Design review of the part built by this model. Coordinates are the model's own, in mm. Coordinates: 2 decimals unless noted, no trailing zeros. Write each loop counter-clockwise with the first axis right and the second up, starting at its lowest first coordinate (ties: lowest second). Pieces come first, ordered by that corner, then holes.
Q1. Add section B-B, the plane x = 4.15. Give the boundary of the cut face in (y, z), plus the area to 3 significant figures.
Q2. To check wall thickness, follow probe 1 along Y at (x, z) = (3.6, -4.45); probe 2 along Y at (x, z) = (3.65, -3.4); probe 3 along Z at (x, y) = (4.65, -2.5). State the ranges of each line that lie inside material, in increasing order.
Q3. Add section A-A, the plane z = -5.45. Give the boundary of the cut face in (x, y).
from build123d import *
from build123d import SkipClean  # not in build123d's __all__

# Parameters (mm, degrees)
F0_W     = 6
F0_H     = 6
F1_DEPTH = 3
F3_ANGLE = 180


with BuildPart() as f1:
    # F0 (on Front) → F1 (new body)
    with BuildSketch(Plane.XZ):
        with Locations((3.4017860889, -4.7885723032)):
            Rectangle(F0_W, F0_H)
    extrude(amount=F1_DEPTH)

    # F2 (on face) → F3 (revolve, cut)
    with BuildSketch(Plane.XZ.offset(3)):
        with BuildLine():
            ThreePointArc((3.4017860889, -6.7885723032), (5.4017860889, -4.7885723032), (3.4017860889, -2.7885723032))
            Line((3.4017860889, -2.7885723032), (3.4017860889, -6.7885723032))
        make_face()
    revolve(axis=Axis((3.4017860889, -3, -4.7885723032), (0, 0, 1)), revolution_arc=F3_ANGLE, mode=Mode.SUBTRACT)

    # F4: F1 across face


with BuildPart() as f1_1:
    add(f1.part, clean=False)
    with SkipClean():  # cleaning this boolean's faces spoils the solid; the shape is the same uncleaned
        add(f1.part.mirror(Plane(origin=(3.4017860889, -3, -4.7885723032), x_dir=(1, 0, 0), z_dir=(0, -1, 0))), clean=False)


solid = f1_1.part
Here are the results:
1. outline: (-6, -7.79) - (0, -7.79) - (0, -1.79) - (-6, -1.79) - close; hole circle Ø3.71 at (-3, -4.79)
1. area: 25.2 mm2
2. probe 1: y = -6 to -4.96, -1.04 to 0
2. probe 2: y = -6 to -4.42, -1.58 to 0
2. probe 3: z = -7.79 to -6.27, -3.31 to -1.79
3. outline: (0.4, -6) - (6.4, -6) - (6.4, 0) - (0.4, 0) - close; hole circle Ø3.77 at (3.4, -3)
